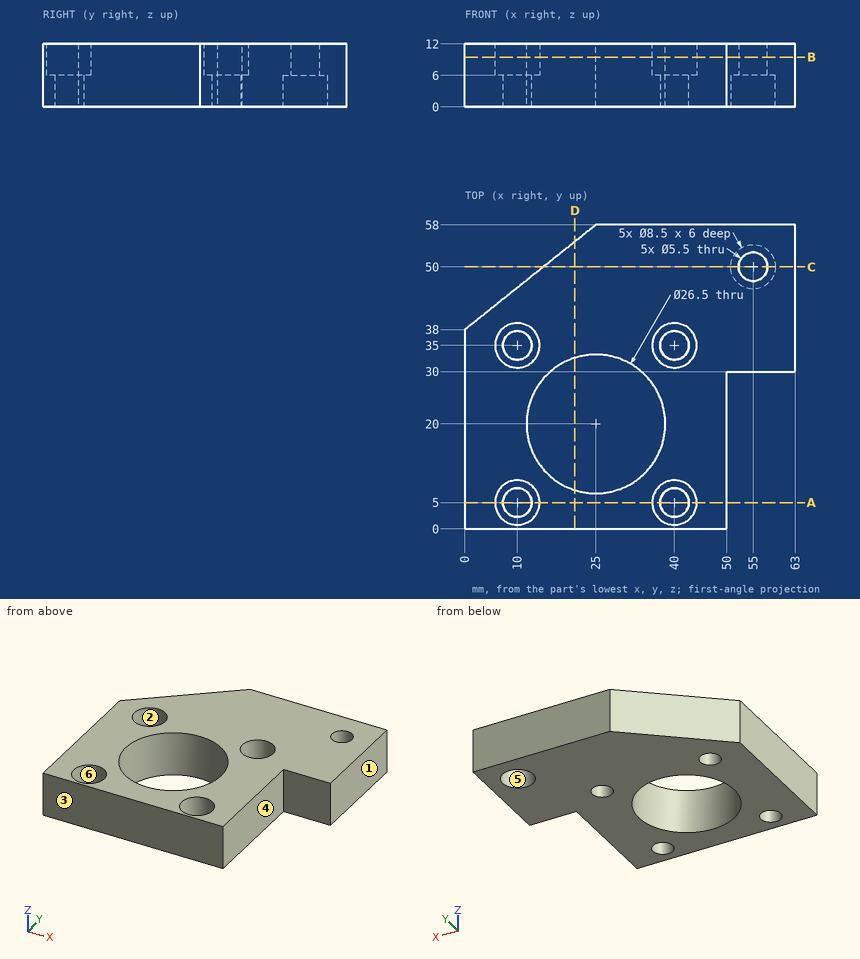
Geometry check sheet. Reference: drawing and pictorial views, mm from the part's lowest x, y, z. A direction names the side the tool comes from. Round coordinates to 2 decimals unless told otherwise and drop trailing zeros. Loops run counter-clockwise (first coordinate to the right, second up) from the corner with the lowest first, then second, coordinate; pieces in that order, holes last. Notation, with made-up numbers: (41, -35.5) - (71, -35.5) arc R27 ccw to (71, -6.5) - close; hole circle Ø1 at (16.5, 25.5). An arc over 180 degrees is marked (long way). One line per question, with ' | ' between items. Start each with the question number.
1. Draft check along Y on the marked faces 1, 2 and 3. Enter one of: released by +Y, released by -Y, zero draft, split by the parting line, or undercut.
2. Cross-section at A-A on y = 5. Record the cut outline in (x, z), then the cut area to 3 significant figures.
3. Scan lines: line 1 (Y direction, x = 40, z = 8.05); line 2 (Y direction, x = 40, z = 3.4); line 3 (X direction, y = 35, z = 2.4). Record each from-to range of solid material in increasing order. Write a range as [from, to].
4. Cross-section at B-B on z = 9.5. Record the cut outline in (x, y).
5. Cross-section at D-D on x = 21. Record the cut outline in (y, z), then the cut area to 3 significant figures.
6. Cross-section at C-C on y = 50. Record the cut outline in (x, z).
7. Depth check by flat-ended pin: pin 1 (2.5 mm diameter, centred on x = 10.5, y = 36.5, fed in from +Z); pin 2 (2.5 mm diameter, centred on x = 57, y = 49, fed in from -Z); pin 3 (6 mm diameter, centred on y = 20, z = 7.5, fed in from +X). Enter the tip coordinate at first touch or a pass-through.
8. Tool access check on the marked faces 4, 5 and 6. Record the directions out of +Z, -Z, +X, -X, +Y, -Y that give a thin tool (end or side, any length) a straight path to the whole face; none if there is none.
Taken from the geometry:
1) face 1: zero draft | face 2: undercut | face 3: released by -Y
2) outline: (0, 0) - (7.25, 0) - (7.25, 6) - (5.75, 6) - (5.75, 12) - (0, 12) - close; (12.75, 0) - (37.25, 0) - (37.25, 6) - (35.75, 6) - (35.75, 12) - (14.25, 12) - (14.25, 6) - (12.75, 6) - close; (42.75, 0) - (50, 0) - (50, 12) - (44.25, 12) - (44.25, 6) - (42.75, 6) - close | area: 432 mm²
3) line 1: [0, 0.75], [9.25, 30.75], [39.25, 58] | line 2: [0, 2.25], [7.75, 32.25], [37.75, 58] | line 3: [0, 7.25], [12.75, 37.25], [42.75, 63]
4) outline: (0, 0) - (50, 0) - (50, 30) - (63, 30) - (63, 58) - (25, 58) - (0, 38) - close; hole circle Ø8.5 at (10, 5); hole circle Ø8.5 at (10, 35); hole circle Ø26.5 at (25, 20); hole circle Ø8.5 at (40, 5); hole circle Ø8.5 at (40, 35); hole circle Ø5.5 at (55, 50)
5) outline: (0, 0) - (7.37, 0) - (7.37, 12) - (0, 12) - close; (32.63, 0) - (54.8, 0) - (54.8, 12) - (32.63, 12) - close | area: 354 mm²
6) outline: (15, 0) - (50.75, 0) - (50.75, 6) - (52.25, 6) - (52.25, 12) - (15, 12) - close; (57.75, 6) - (59.25, 6) - (59.25, 0) - (63, 0) - (63, 12) - (57.75, 12) - close
7) pin 1: z = 6 | pin 2: z = 6 | pin 3: x = 50
8) face 4: +Z, -Z, +X, -Y | face 5: -Z | face 6: +Z
